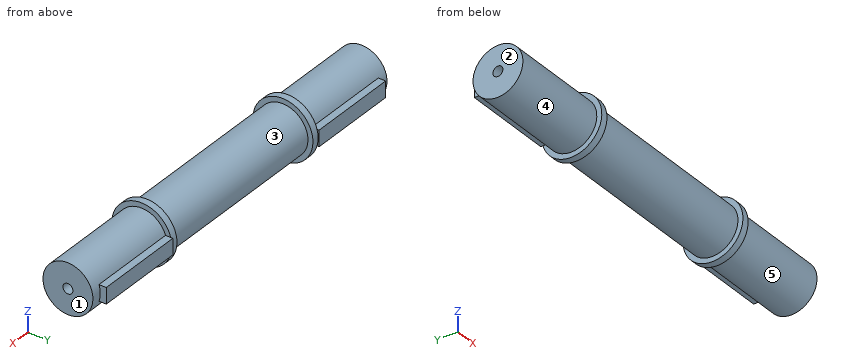
from build123d import *

# Parameters (mm, degrees)
CROQUIS1_R              = 12.5
SALIENTE_EXTRUIR1_DEPTH = 99.5
CROQUIS2_R              = 15
SALIENTE_EXTRUIR2_DEPTH = 3.5
CROQUIS4_W              = 8
CROQUIS4_H              = 3.657280718
SALIENTE_EXTRUIR3_DEPTH = 45
SALIENTE_EXTRUIR4_START = 99
CROQUIS4_2_W            = 8
CROQUIS4_2_H            = 3.657280718
SALIENTE_EXTRUIR4_DEPTH = 45
SALIENTE_EXTRUIR5_START = -92
CROQUIS2_2_R            = 15
SALIENTE_EXTRUIR5_DEPTH = 3.5
TALADRO_ROSCADO_M61_D   = 5


with BuildPart() as part:
    # Croquis1 → Saliente-Extruir1 (new body, symmetric)
    with BuildSketch(Plane(origin=(0, 0, 0), x_dir=(0, 0, -1), z_dir=(1, 0, 0))):
        Circle(CROQUIS1_R)
    extrude(amount=SALIENTE_EXTRUIR1_DEPTH, both=True)

    # Croquis2 → Saliente-Extruir2 (add)
    with BuildSketch(Plane(origin=(46, 0, 0), x_dir=(0, 0, -1), z_dir=(1, 0, 0))):
        Circle(CROQUIS2_R)
    extrude(amount=SALIENTE_EXTRUIR2_DEPTH)

    # Croquis4 → Saliente-Extruir3 (add)
    with BuildSketch(Plane.ZY.offset(-49.5)):
        with Locations((0, 13.671359641)):
            Rectangle(CROQUIS4_W, CROQUIS4_H)
    extrude(amount=-SALIENTE_EXTRUIR3_DEPTH)

    # Croquis4<2> → Saliente-Extruir4 (add)
    with BuildSketch(Plane.ZY.offset(-49.5).offset(SALIENTE_EXTRUIR4_START)):
        with Locations((0, 13.671359641)):
            Rectangle(CROQUIS4_2_W, CROQUIS4_2_H)
    extrude(amount=SALIENTE_EXTRUIR4_DEPTH)

    # Croquis2<2> → Saliente-Extruir5 (add)
    with BuildSketch(Plane(origin=(46, 0, 0), x_dir=(0, 0, -1), z_dir=(1, 0, 0)).offset(SALIENTE_EXTRUIR5_START)):
        Circle(CROQUIS2_2_R)
    extrude(amount=-SALIENTE_EXTRUIR5_DEPTH)

    # Taladro roscado M61 (through all)
    with Locations(Plane(origin=(99.5, 0, 0), x_dir=(0, 0, -1), z_dir=(1, 0, 0))):
        with Locations((0, 0)):
            Hole(TALADRO_ROSCADO_M61_D / 2)


solid = part.part
Input: part model. Units: mm. Frame: model coordinates. Face numbers are marked on the shaded views. A direction names the side the tool comes from. Give positions to 0.01 mm unless a question says otherwise; leave off trailing zeros. Order: outer loops, then holes, each group sorted by start corner. A loop starts at its lowest first (then second) coordinate and runs counter-clockwise, first axis right, second up. Notation, with made-up numbers: (14, 16.25) - (54, 16.25) arc R10 cw to (54, 25.25) - close; hole circle Ø5 at (-29.5, 1). An arc over 180 degrees is marked (long way). Answer as a JSON object with one key per item and string values. Group by question number.
Q1. Line query: probe 1 along Y at (x, z) = (-33.5, 0); probe 2 along X at (y, z) = (13, -1); probe 3 along X at (y, z) = (13, 5). Output: solid intervals per line, ascending.
Q2. First-contact query: pin 1 Ø1.5 at (x, z) = (-40, -10) entering from +Y; pin 2 Ø0.5 at (y, z) = (14.5, -0.5) entering from +X; pin 3 Ø1.1 at (x, y) = (-82, 14) entering from -Z; pin 4 Ø9 at (y, z) = (-1, 0) entering from -X. Flat tips, straight axial feed; report the tip coordinate or a pass-through.
Q3. Cut plane D-D, the plane x = 34. Output: boundary loops of the cut face in (y, z).
Q4. Cut plane C-C, the plane x = -52. Output: boundary loops of the cut face in (y, z).
Q5. Cut plane B-B, the plane y = 0. Output: boundary loops of the cut face in (x, z), then the cut area to 4 significant figures.
Q6. Mould query, pull axis X, two halves, no side actions, for the marked faces 1, 2 and 3. Classes: pulls with the +X half, pulls with the -X half, needs draft (parallel to the pull), parting line crosses it, or undercut.
Q7. Set-up query: the marked faces 4 and 5. Return all of +Z, -Z, +X, -X, +Y, -Y with unobstructed straight access to the full face (end or side cutting, diameter ignored); none if empty.
Q8. Cut plane A-A, the plane z = 0. Output: boundary loops of the cut face in (x, y).
Results:
{
 "1": {"probe 1": "-12.5 to -2.5, 2.5 to 12.5", "probe 2": "-94.5 to -46, 46 to 94.5", "probe 3": "-49.5 to -46, 46 to 49.5"},
 "2": {"pin 1": "y = 8.41", "pin 2": "x = 94.5", "pin 3": "z = -4", "pin 4": "x = -99.5"},
 "3": {"outline": "circle Ø25 at (0, 0); hole circle Ø5 at (0, 0)"},
 "4": {"outline": "(11.84, -4) - (15.5, -4) - (15.5, 4) - (11.84, 4) arc R12.5 ccw (long way) to start; hole circle Ø5 at (0, 0)"},
 "5": {"outline": "(-99.5, -12.5) - (-49.5, -12.5) - (-49.5, -15) - (-46, -15) - (-46, -12.5) - (46, -12.5) - (46, -15) - (49.5, -15) - (49.5, -12.5) - (99.5, -12.5) - (99.5, -2.5) - (-99.5, -2.5) - close; (-99.5, 2.5) - (99.5, 2.5) - (99.5, 12.5) - (49.5, 12.5) - (49.5, 15) - (46, 15) - (46, 12.5) - (-46, 12.5) - (-46, 15) - (-49.5, 15) - (-49.5, 12.5) - (-99.5, 12.5) - close", "area": "4,015 mm^2"},
 "6": {"face 1": "pulls with the +X half", "face 2": "pulls with the -X half", "face 3": "undercut"},
 "7": {"face 4": "-X", "face 5": "+X"},
 "8": {"outline": "(-99.5, -12.5) - (-49.5, -12.5) - (-49.5, -15) - (-46, -15) - (-46, -12.5) - (46, -12.5) - (46, -15) - (49.5, -15) - (49.5, -12.5) - (99.5, -12.5) - (99.5, -2.5) - (-99.5, -2.5) - close; (-99.5, 2.5) - (99.5, 2.5) - (99.5, 12.5) - (94.5, 12.5) - (94.5, 15.5) - (49.5, 15.5) - (49.5, 15) - (46, 15) - (46, 12.5) - (-46, 12.5) - (-46, 15) - (-49.5, 15) - (-49.5, 15.5) - (-94.5, 15.5) - (-94.5, 12.5) - (-99.5, 12.5) - close"}
}
